```python
from build123d import *

# Parameters (mm, degrees)
F1_DEPTH = 63.5
F2_DEPTH = 7.9375
F3_DEPTH = 25.4
F5_R     = 6.35


with BuildPart() as f1:
    # F0 (on Front) → F1 (new body, symmetric)
    with BuildSketch(Plane.XZ):
        Polygon((-41.275, 9.525), (-41.275, -9.525), (41.275, -9.525), (41.275, 9.525), (22.225, 9.525), align=None)
    extrude(amount=F1_DEPTH, both=True)

    # F0 (on Front) → F2 (join, symmetric)
    with BuildSketch(Plane.XZ):
        with BuildLine():
            add(Edge.make_bspline(
                [(-41.275, 9.525), (-41.15331158, 43.5455983009), (15.5951323603, 60.6045840668), (54.8853746059, 61.8517006395)],
                knots=[0, 0, 0, 0, 109.2519553894, 109.2519553894, 109.2519553894, 109.2519553894], degree=3))
            Line((-41.275, 9.525), (22.225, 9.525))
            Line((22.225, 9.525), (22.225, 27.0002))
            ThreePointArc((22.225, 27.0002), (31.666204493, 50.8818203712), (54.8853746059, 61.8517006395))
        make_face()
    extrude(amount=F2_DEPTH, both=True)

    # F0 (on Front) → F3 (join, symmetric)
    with BuildSketch(Plane.XZ):
        Polygon((98.005393815, 61.9252), (72.4958287168, 61.9252), (72.4958287168, 42.8752), (97.9177884222, 42.8752), align=None)
        with BuildLine():
            Line((22.225, 9.525), (41.275, 9.525))
            Line((41.275, 9.525), (41.275, 27.0002))
            ThreePointArc((41.275, 27.0002), (45.9246798487, 38.2255201513), (57.15, 42.8752))
            Line((57.15, 42.8752), (72.4958287168, 42.8752))
            Line((72.4958287168, 42.8752), (72.4958287168, 61.9252))
            Line((72.4958287168, 61.9252), (59.1482142662, 61.9252))
            add(Edge.make_bspline(
                [(54.8853746059, 61.8517006395), (56.3311922229, 61.8975925202), (57.7533693148, 61.92207321), (59.1482142662, 61.9252)],
                knots=[109.2519553894, 109.2519553894, 109.2519553894, 109.2519553894, 113.2722513399, 113.2722513399, 113.2722513399, 113.2722513399], degree=3))
            ThreePointArc((54.8853746059, 61.8517006395), (31.666204493, 50.8818203712), (22.225, 27.0002))
            Line((22.225, 27.0002), (22.225, 9.525))
        make_face()
    extrude(amount=F3_DEPTH, both=True)

    # F0 (on Front) → F4 (revolve)
    with BuildSketch(Plane.XZ):
        Polygon((98.0272367597, 66.675), (98.005393815, 61.9252), (97.9177884222, 42.8752), (97.8958287168, 38.100010092), (123.2958287168, 38.100010092), (123.2958287168, 66.675), align=None)
    revolve(axis=Axis((97.9615327382, 0, 52.387505046), (0.0045986597, 0, 0.9999894261)))

    # F5
    f5_edges = [f1.edges().sort_by_distance(p)[0] for p in [
        (-41.275, -63.5, 0),
        (41.275, -63.5, 0),
        (41.275, 63.5, 0),
        (-41.275, 63.5, 0),
    ]]
    fillet(f5_edges, radius=F5_R)


solid = f1.part
```
The listing builds one solid part. Answer for the finished solid, in the listing's coordinates (mm). A direction names the side the tool comes from. Coordinates: 2 decimals unless noted, no trailing zeros. Write each loop counter-clockwise with the first axis right and the second up, starting at its lowest first coordinate (ties: lowest second). Pieces come first, ordered by that corner, then holes.
Q1. Section B-B, the plane y = 43.5 is taken. Write down the section's boundary in (x, z) (3 decimals).
Returned:
outline: (-41.275, -9.525) - (41.275, -9.525) - (41.275, 9.525) - (-41.275, 9.525) - close
Q2. Section A-A, the plane z = 0 is taken. Write down the section's boundary in (x, y) (3 decimals), then the cut area to 3 significant figures.
Returned:
outline: (-41.275, -57.15) arc R6.35 ccw to (-34.925, -63.5) - (34.925, -63.5) arc R6.35 ccw to (41.275, -57.15) - (41.275, 57.15) arc R6.35 ccw to (34.925, 63.5) - (-34.925, 63.5) arc R6.35 ccw to (-41.275, 57.15) - close
area: 10,400 mm2
Q3. Which of the six approach directions +Z, -Z, +X, -X, +Y, -Y give full straight-line access (tool end or side, diameter ignored) to faces 1 (the cylindrical face through (31.92, -16.79, 51.15)), 2 (the flat face through (-3, 7.938, 30)), 3 (the flat face through (41.275, -1, 4))?
Returned:
face 1: +Z, -X, -Y
face 2: +Z, -X, +Y
face 3: -Z, +X, +Y, -Y
Q4. Find the intervals of material crossed by line 1 along X through (y, z) = (-47, 4.5) (3 decimals); line 2 along Z through (x, y) = (-3, -48) (3 decimals); line 3 along Y through (x, z) = (90.5, 44), in increasing order.
Returned:
line 1: x = -41.275 to 41.275
line 2: z = -9.525 to 9.525
line 3: y = -25.4 to 25.4
Q5. Given P1, Ø18.5, axis at y = 28.5, z = 4.5, coming from the +X side (3 decimals); P2, Ø5, axis at y = 14.5, z = 21, coming from the -X side (3 decimals); P3, Ø1.5, axis at y = 15, z = 52.5, coming from the +X side, each flat-ended and moving along its own axis, determine where each tip first touches the part or whether it passes through.
Returned:
P1: stops at x = 41.275
P2: stops at x = 22.225
P3: stops at x = 118.91
